Autodesk Inventor part; units mm, degrees
ref_plane "YZ Plane" through (0, 0, 0) normal (1, 0, 0) x (0, 1, 0)
ref_plane "XZ Plane" through (0, 0, 0) normal (0, 1, 0) x (-1, 0, 0)
ref_plane "XY Plane" through (0, 0, 0) normal (0, 0, 1) x (1, 0, 0)
sketch "Sketch1" plane through (0, 0, 0) normal (0, 0, 1) x (1, 0, 0)
  line L0 (0, 0) -> (35.3316, 0)
  line L1 (0, 0) -> (16.5, 0)
  line L2 (16.5, 0) -> (16.5, 6)
  line L3 (16.5, 6) -> (0, 6)
  line L4 (0, 6) -> (0, 0)
  dimension "d0" = 16.5
  dimension "d1" = 6
extrude "Extrusion1" add sketch "Sketch1" along normal blind 1.75
sketch "Sketch2" plane through (0, 0, 1.75) normal (0, 0, 1) x (1, 0, 0)
  line L0 (0, 0) -> (16.5, 0)
  line L1 (16.5, 0) -> (16.5, 6)
  line L2 (16.5, 6) -> (0, 6)
  line L3 (0, 6) -> (0, 0)
  line L4 (8.25, 6) -> (8.25, 0) construction
  circle A0 centre (8.25, 3) radius 3.15
  dimension "d4" = 6.3
extrude "Extrusion2" add sketch "Sketch2" along normal blind 7.5 contours A0 L2 L0 | L0 A0 | A0 L2
sketch "Sketch3" plane through (0, 0, 0) normal (0, 0, -1) x (-1, 0, 0)
  line L0 (0, 0) -> (-16.5, 0)
  line L1 (0, 6) -> (0, 0)
  line L2 (-16.5, 6) -> (0, 6)
  line L3 (-16.5, 0) -> (-16.5, 6)
  line L4 (-8.25, 6) -> (-8.25, 0) construction
  circle A0 centre (-8.25, 3) radius 2.5
  dimension "d7" = 5
extrude "Extrusion3" add sketch "Sketch3" along normal blind 13 contours A0
properties part number "SMA whip end"
Geometry check sheet. Reference: the model listing, model coordinates, mm. A direction names the side the tool comes from. Round coordinates to 2 decimals unless told otherwise and drop trailing zeros. Order: outer loops, then holes, each group sorted by start corner. A loop starts at its lowest first (then second) coordinate and runs counter-clockwise, first axis right, second up. Notation, with made-up numbers: M -26.75,75.5 L 13.25,75.5 A26 ccw 13.25,89.5 Z; hole C 22,-14 d6. An arc over 180 degrees is marked long. Answer in a Markdown table with one row per item. Add a question column.
Item 1: Set-up check for faces 1 (the face through (0, 3, 1)), 2 (the face through (10.748, 2.89, -6.409)), 3 (the face through (5.75, 4.917, 5.448)): record each of +Z, -Z, +X, -X, +Y, -Y from which the full face is reachable in a straight line by a thin tool's end or side.
Item 2: Sectioned sample at C-C, the plane z = -8.75. Enter the section's corners in (x, y).
Item 3: Sectioned sample at B-B, the plane x = 8.25. Enter the section's corners in (y, z), plus the area to 3 significant figures.
Item 4: Sectioned sample at A-A, the plane y = 3. Enter the section's corners in (x, z).
Item 5: Sectioned sample at D-D, the plane x = 4. Enter the section's corners in (y, z), plus the area to 3 significant figures.
Item 6: Depth check by flat-ended pin: pin 1 Ø1 at (x, y) = (5.5, 5.5) entering from +Z; pin 2 Ø3 at (y, z) = (2.5, -5) entering from +X; pin 3 Ø1.9 at (x, z) = (5.5, 0.5) entering from +Y. Enter the tip coordinate at first touch or a pass-through.
Item 7: Material ranges on L1, parallel to Z at x = 14, y = 3.25; L2, parallel to Z at x = 11, y = 4; L3, parallel to Y at x = 3, z = 1.25, recorded low to high. Write a range as [from, to].
Filled in:
| question | item | result |
|---|---|---|
| 1 | face 1 | +Z, -Z, -X, +Y, -Y |
| 1 | face 2 | -Z |
| 1 | face 3 | +Z |
| 2 | outline | C 8.25,3 d5 |
| 3 | outline | M -0.15,1.75 L 0,1.75 L 0,0 L 0.5,0 L 0.5,-13 L 5.5,-13 L 5.5,0 L 6,0 L 6,1.75 L 6.15,1.75 L 6.15,9.25 L -0.15,9.25 Z |
| 3 | area | 123 mm² |
| 4 | outline | M 0,0 L 5.75,0 L 5.75,-13 L 10.75,-13 L 10.75,0 L 16.5,0 L 16.5,1.75 L 11.4,1.75 L 11.4,9.25 L 5.1,9.25 L 5.1,1.75 L 0,1.75 Z |
| 5 | outline | M 0,0 L 6,0 L 6,1.75 L 0,1.75 Z |
| 5 | area | 10.5 mm² |
| 6 | pin 1 | stops at z = 1.75 |
| 6 | pin 2 | stops at x = 10.75 |
| 6 | pin 3 | stops at y = 6 |
| 7 | L1 | z = [0, 1.75] |
| 7 | L2 | z = [0, 9.25] |
| 7 | L3 | y = [0, 6] |
